Check sheet for the modelled part. Datum: model origin and axes. Units: mm. Face numbers are marked on the shaded views. Round coordinates to 2 decimals unless told otherwise and drop trailing zeros. Write each loop counter-clockwise with the first axis right and the second up, starting at its lowest first coordinate (ties: lowest second). Pieces come first, ordered by that corner, then holes.
from build123d import *

# Parameters (mm, degrees)
BOSS_EXTRUDE1_DEPTH = 10
FILLET1_R           = 3
FILLET2_R           = 1.72427
FILLET3_R           = 1.72427


with BuildPart() as part:
    # Sketch1 → Boss-Extrude1 (new body)
    with BuildSketch(Plane(origin=(0, 0, 0), x_dir=(1, 0, 0), z_dir=(0, 1, 0))):
        Polygon((0, -16.5), (0, -20), (-20, -20), (-20, 20), (0, 20), (0, 16.5), (-17, 17), (-17, -17), align=None)
    extrude(amount=BOSS_EXTRUDE1_DEPTH)

    # Fillet1
    fillet1_edges = [part.edges().sort_by_distance(p)[0] for p in [
        (-20, 5, -20),
        (-20, 5, 20),
    ]]
    fillet(fillet1_edges, radius=FILLET1_R)

    # Fillet2
    fillet2_edges = [part.edges().sort_by_distance(p)[0] for p in [
        (0, 5, 16.5),
        (0, 5, 20),
    ]]
    fillet(fillet2_edges, radius=FILLET2_R)

    # Fillet3
    fillet3_edges = [part.edges().sort_by_distance(p)[0] for p in [
        (0, 5, -20),
        (0, 5, -16.5),
    ]]
    fillet(fillet3_edges, radius=FILLET3_R)


solid = part.part
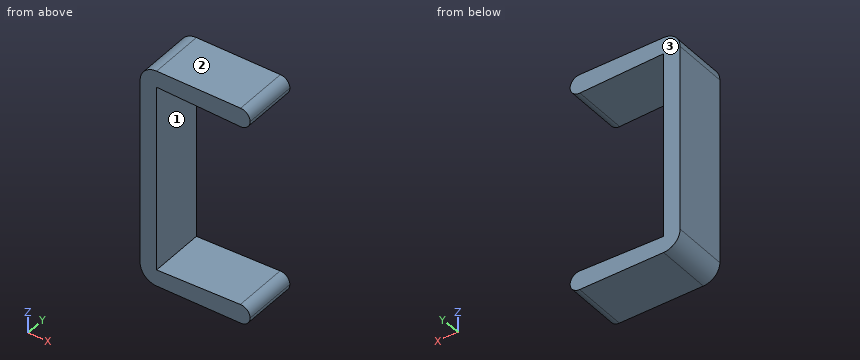
1. Scan lines: line 1 along Z through (x, y) = (-2, 4); line 2 along X through (y, z) = (4.25, 16.5); line 3 along Z through (x, y) = (-8.5, 8). Record each from-to range of solid material in increasing order.
2. Release check for a two-part mould opening along Z. For the marked faces 1, 2 and 3 record: released by +Z, released by -Z, zero draft, split by the parting line, or undercut.
3. Sectioned sample at C-C, the plane z = -11. Enter the section's corners in (x, y), plus the area to 3 significant figures.
4. Sectioned sample at B-B, the plane y = 7.75. Enter the section's corners in (x, z).
5. Sectioned sample at A-A, the plane x = -8.5. Enter the section's corners in (y, z), plus the area to 3 significant figures.
6. Sectioned sample at D-D, the plane x = -3.25. Enter the section's corners in (y, z).
7. Go/stop test with a flat-tipped pin: pin 1 (10 mm diameter, centred on x = -16.5, z = -11, fed in from +Y). Record where the tip stops, or that it passes through.
Computed values:
1. line 1: z = -20 to -16.56, 16.56 to 20
1. line 2: x = -20 to -17
1. line 3: z = -20 to -16.75, 16.75 to 20
2. face 1: undercut
2. face 2: released by +Z
2. face 3: zero draft
3. outline: (-20, 0) - (-17, 0) - (-17, 10) - (-20, 10) - close
3. area: 30.0 mm2
4. outline: (-20, -17) arc R3 ccw to (-17, -20) - (-1.72, -20) arc R1.72 ccw (long way) to (-1.77, -16.55) - (-17, -17) - (-17, 17) - (-1.77, 16.55) arc R1.72 ccw (long way) to (-1.72, 20) - (-17, 20) arc R3 ccw to (-20, 17) - close
5. outline: (0, -20) - (10, -20) - (10, -16.75) - (0, -16.75) - close; (0, 16.75) - (10, 16.75) - (10, 20) - (0, 20) - close
5. area: 65.0 mm2
6. outline: (0, -20) - (10, -20) - (10, -16.6) - (0, -16.6) - close; (0, 16.6) - (10, 16.6) - (10, 20) - (0, 20) - close
7. pin 1: stops at y = 10
